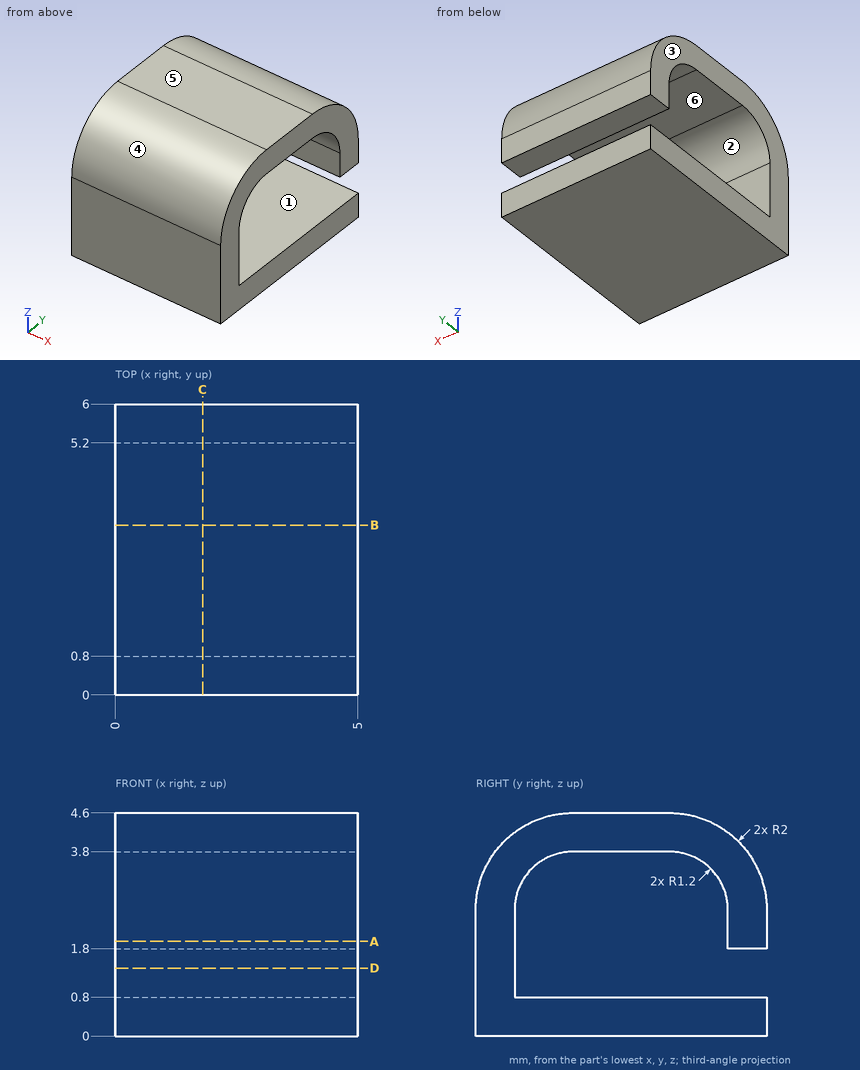
Geometry check sheet. Reference: drawing and pictorial views, mm from the part's lowest x, y, z. A direction names the side the tool comes from. Coordinates: 2 decimals unless noted, no trailing zeros. Loops run counter-clockwise (first coordinate to the right, second up) from the corner with the lowest first, then second, coordinate; pieces in that order, holes last. Notation, with made-up numbers: (-7, 39.5) -> (51, 39.5) arc R14 cw to (51, 57.5) -> close; hole circle Ø6 at (48, -1). An arc over 180 degrees is marked (long way). Write item = value, one per line. Start each with the question number.
1. Section check B-B on y = 3.5. Record the cut outline in (x, z).
2. Material ranges on line 1 (Z direction, x = 1.35, y = 4); line 2 (Y direction, x = 4.15, z = 2.05); line 3 (Y direction, x = 0.95, z = 2.95), recorded low to high.
3. Section check C-C on x = 1.8. Record the cut outline in (y, z), then the cut area to 3 significant figures.
4. Tool access check on the marked faces 1, 2 and 3. Record the directions out of +Z, -Z, +X, -X, +Y, -Y that give a thin tool (end or side, any length) a straight path to the whole face; none if there is none.
5. Section check A-A on z = 1.95. Record the cut outline in (x, y).
6. Draft check along Y on the marked faces 4, 5 and 6. Enter one of: released by +Y, released by -Y, zero draft, split by the parting line, or undercut.
7. Section check D-D on z = 1.4. Record the cut outline in (x, y), then the cut area to 3 significant figures.
Responses:
q1.outline = (0, 0) -> (5, 0) -> (5, 0.8) -> (0, 0.8) -> close; (0, 3.8) -> (5, 3.8) -> (5, 4.6) -> (0, 4.6) -> close
q2.line_1 = 0 to 0.8, 3.8 to 4.6
q2.line_2 = 0 to 0.8, 5.2 to 6
q2.line_3 = 0.03 to 0.85, 5.15 to 5.97
q3.outline = (0, 0) -> (6, 0) -> (6, 0.8) -> (0.8, 0.8) -> (0.8, 2.6) arc R1.2 cw to (2, 3.8) -> (4, 3.8) arc R1.2 cw to (5.2, 2.6) -> (5.2, 1.8) -> (6, 1.8) -> (6, 2.6) arc R2 ccw to (4, 4.6) -> (2, 4.6) arc R2 ccw to (0, 2.6) -> close
q3.area = 12.5 mm2
q4.face_1 = +X, -X, +Y
q4.face_2 = +X, -X
q4.face_3 = +Z, -Z, -X, +Y, -Y
q5.outline = (0, 0) -> (5, 0) -> (5, 0.8) -> (0, 0.8) -> close; (0, 5.2) -> (5, 5.2) -> (5, 6) -> (0, 6) -> close
q6.face_4 = released by -Y
q6.face_5 = zero draft
q6.face_6 = undercut
q7.outline = (0, 0) -> (5, 0) -> (5, 0.8) -> (0, 0.8) -> close
q7.area = 4.00 mm2
